The drawing under review shows one solid part. Ordinate dimensions are in mm from its lowest x, y, z. Give positions to 0.01 mm unless a question says otherwise; leave off trailing zeros. Order: outer loops, then holes, each group sorted by start corner. A loop starts at its lowest first (then second) coordinate and runs counter-clockwise, first axis right, second up. Notation, with made-up numbers: (17.25, -9.75) - (38.25, -9.75) arc R18 ccw to (38.25, -2.75) - close; hole circle Ø2 at (76, 84). An arc over 180 degrees is marked (long way). Use CSV: the item, a comma, the result in double quotes.
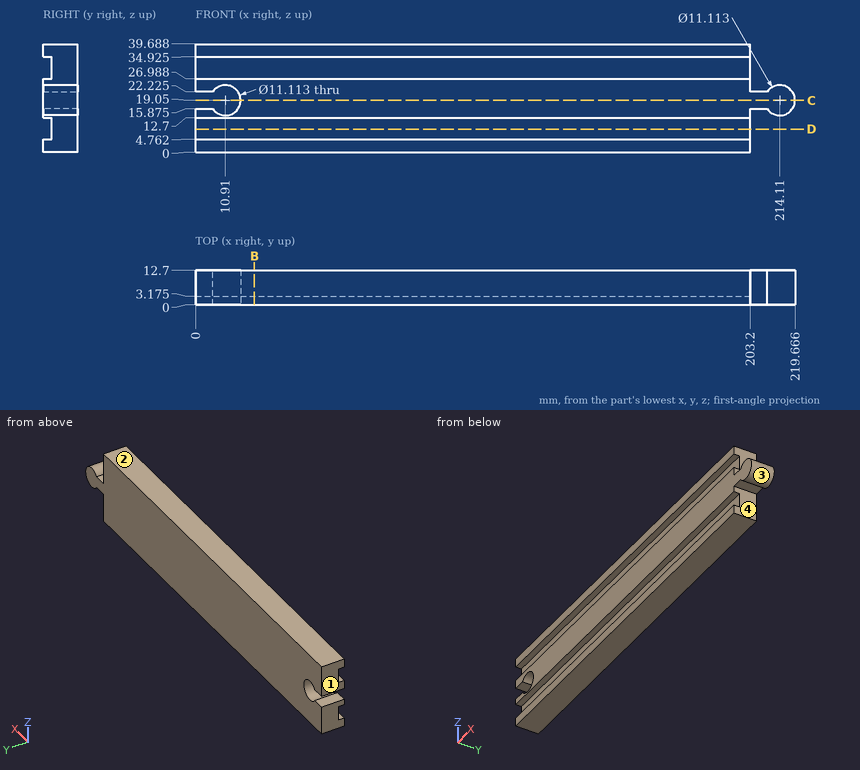
Item 1: Mouldability with a two-part tool opening along X and no side actions: class the marked faces 1, 2, 3 and 4 as pulls with the +X half, pulls with the -X half, needs draft (parallel to the pull), parting line crosses it, or undercut.
Results list:
face 1,"pulls with the -X half"
face 2,"needs draft"
face 3,"undercut"
face 4,"undercut"
Item 2: Take a section at C-C, the plane z = 19.05. Give the boundary of the cut face in (x, y) (1 decimal).
Results list:
outline,"(16.5, 0) - (219.7, 0) - (219.7, 12.7) - (16.5, 12.7) - close"
Item 3: Clearance check with flat-ended pins moving along their axes: pin 1 (5 mm diameter, centred on x = 207.5, y = 7.5, fed in from -Z); pin 2 (3 mm diameter, centred on y = 8, z = 35, fed in from +X); pin 3 (2.5 mm diameter, centred on x = 125.5, z = 30.5, fed in from -Y) (1 decimal). State where each tip first meets the part, or that it passes through.
Results list:
pin 1,"stops at z = 15.31"
pin 2,"stops at x = 203.2"
pin 3,"stops at y = 3.2"
Item 4: Take a section at D-D, the plane z = 8.5. Give the boundary of the cut face in (x, y) (1 decimal).
Results list:
outline,"(0, 3.2) - (203.2, 3.2) - (203.2, 12.7) - (0, 12.7) - close"
Item 5: Wall thickness on L1, parallel to Z at x = 141, y = 1.25 (1 decimal); L2, parallel to X at y = 11.25, z = 15 (1 decimal); L3, parallel to Y at x = 46, z = 32.5 (1 decimal): over which ranges is each line inside the solid? List them lowest first.
Results list:
L1,"z = 0 to 4.8, 12.7 to 27, 34.9 to 39.7"
L2,"x = 0 to 7.1, 14.7 to 203.2, 210.3 to 217.9"
L3,"y = 3.2 to 12.7"
Item 6: Take a section at B-B, the plane x = 21.5. Give the boundary of the cut face in (y, z) (1 decimal), and give its area (3 significant figures).
Results list:
outline,"(0, 0) - (12.7, 0) - (12.7, 39.7) - (0, 39.7) - (0, 34.9) - (3.2, 34.9) - (3.2, 27) - (0, 27) - (0, 12.7) - (3.2, 12.7) - (3.2, 4.8) - (0, 4.8) - close"
area,"454 mm2"
